```python
from build123d import *

# Parameters (mm, degrees)
F0_R     = 1.905
F1_DEPTH = 2.54
F2_W     = 63.5
F2_H     = 6.35
F3_DEPTH = 12.7
F4_R     = 1.27
F5_R     = 1.27


with BuildPart() as f1:
    # F0 (on Top) → F1 (new body)
    with BuildSketch(Plane.XY):
        Polygon((5.08, 25.4), (5.08, 0), (68.58, 0), (68.58, 25.4), (58.42, 25.4), (58.42, 15.24), (53.34, 10.16), (20.32, 10.16), (15.24, 15.24), (15.24, 25.4), align=None)
        with Locations((10.16, 19.05)):
            Circle(F0_R, mode=Mode.SUBTRACT)
        with Locations((63.5, 19.05)):
            Circle(F0_R, mode=Mode.SUBTRACT)
    extrude(amount=F1_DEPTH)

    # F2 (on face) → F3 (join)
    with BuildSketch(Plane.XY.offset(2.54)):
        with Locations((36.83, 3.175)):
            Rectangle(F2_W, F2_H)
    extrude(amount=F3_DEPTH)

    # F4
    f4_edges = [f1.edges().sort_by_distance(p)[0] for p in [
        (36.83, 0, 15.24),
        (36.83, 6.35, 15.24),
        (68.58, 0, 7.62),
        (68.58, 6.35, 8.89),
        (68.58, 3.175, 15.24),
        (5.08, 3.175, 15.24),
        (5.08, 0, 7.62),
        (5.08, 6.35, 8.89),
    ]]
    fillet(f4_edges, radius=F4_R)

    # F5
    f5_edges = [f1.edges().sort_by_distance(p)[0] for p in [
        (68.58, 25.4, 1.27),
        (58.42, 25.4, 1.27),
        (15.24, 25.4, 1.27),
        (5.08, 25.4, 1.27),
    ]]
    fillet(f5_edges, radius=F5_R)


solid = f1.part
```
Source: CAD feature listing. Evaluate the final solid. Frame: model axes, mm. A direction names the side the tool comes from. Round coordinates to 2 decimals unless told otherwise and drop trailing zeros. Loops run counter-clockwise (first coordinate to the right, second up) from the corner with the lowest first, then second, coordinate; pieces in that order, holes last. Notation, with made-up numbers: M 15,83 L 26,83 A10 cw 26,98 Z; hole C 82.25,76 d1. An arc over 180 degrees is marked long. Use a Markdown table: item, result. Add a question column.
1. Reachability of faces 1 (the flat face through (36, 6.35, 8)), 2 (the cylindrical face through (5.442, 5.968, 8.335)), 3 (the cylindrical face through (14.858, 25.038, 1.288)) from +Z, -Z, +X, -X, +Y, -Y: full face, straight path, thin tool, end or side. Return the list, or none.
2. Section query C-C on z = 13.25. Return the cut outline in (x, y), then the cut area to 3 significant figures.
3. Mould query, pull axis Y, two halves, no side actions, for faces 4 (the cylindrical face through (8.65, 17.89, 1.25)), 5 (the cylindrical face through (68.198, 0.362, 7.083)), 6 (the flat face through (29, 9, 2.54)), 7 (the cylindrical face through (37.257, 5.988, 14.858)). Classes: pulls with the +Y half, pulls with the -Y half, needs draft (parallel to the pull), parting line crosses it, or undercut.
4. Section query D-D on x = 19. Return the cut outline in (y, z), then the cut area to 3 significant figures.
5. Contact query for flat-ended pins moving along their axis: P1, Ø1.5, axis at y = 21.5, z = 4, coming from the -X side; P2, Ø2, axis at x = 33, z = 1.5, coming from the +Y side; P3, Ø4.5, axis at x = 63.5, y = 19.05, coming from the +Z side; P4, Ø5.5, axis at x = 37, z = 6, coming from the +Y side. Output: stop coordinate, or through.
6. Section query A-A on y = 19.05. Return the cut outline in (x, z) (3 decimals), then the cut area to 3 significant figures.
7. Section query B-B on x = 63.5. Return the cut outline in (y, z) (3 decimals).
8. Line query: line 1 (Y direction, x = 10.16, z = 2.05) (3 decimals); line 2 (Z direction, x = 9.5, y = 12.25); line 3 (Y direction, x = 64, z = 3.75). Output: solid intervals per line, ascending.
Reported:
| question | item | result |
|---|---|---|
| 1 | face 1 | +Z, +X, -X, +Y |
| 1 | face 2 | +Z, -X, +Y |
| 1 | face 3 | +Z, -Z, +Y |
| 2 | outline | M 5.08,1.27 A1.27 ccw 6.35,0 L 67.31,0 A1.27 ccw 68.58,1.27 L 68.58,5.08 A1.27 ccw 67.31,6.35 L 6.35,6.35 A1.27 ccw 5.08,5.08 Z |
| 2 | area | 402 mm² |
| 3 | face 4 | undercut |
| 3 | face 5 | pulls with the -Y half |
| 3 | face 6 | needs draft |
| 3 | face 7 | pulls with the +Y half |
| 4 | outline | M 0,0 L 11.48,0 L 11.48,2.54 L 6.35,2.54 L 6.35,13.97 A1.27 ccw 5.08,15.24 L 1.27,15.24 A1.27 ccw 0,13.97 Z |
| 4 | area | 109 mm² |
| 5 | P1 | passes through |
| 5 | P2 | stops at y = 10.16 |
| 5 | P3 | stops at z = 2.54 |
| 5 | P4 | stops at y = 6.35 |
| 6 | outline | M 5.08,0 L 8.255,0 L 8.255,2.54 L 5.08,2.54 Z; M 12.065,0 L 15.24,0 L 15.24,2.54 L 12.065,2.54 Z; M 58.42,0 L 61.595,0 L 61.595,2.54 L 58.42,2.54 Z; M 65.405,0 L 68.58,0 L 68.58,2.54 L 65.405,2.54 Z |
| 6 | area | 32.3 mm² |
| 7 | outline | M 0,0 L 17.145,0 L 17.145,2.54 L 6.35,2.54 L 6.35,13.97 A1.27 ccw 5.08,15.24 L 1.27,15.24 A1.27 ccw 0,13.97 Z; M 20.955,0 L 25.4,0 L 25.4,2.54 L 20.955,2.54 Z |
| 8 | line 1 | y = 0 to 17.145, 20.955 to 25.4 |
| 8 | line 2 | z = 0 to 2.54 |
| 8 | line 3 | y = 0 to 6.35 |
